Job drawing, mm, ordinate dimensions from the low corner. One solid piece. Coordinates: 2 decimals unless noted, no trailing zeros. Loops run counter-clockwise (first coordinate to the right, second up) from the corner with the lowest first, then second, coordinate; pieces in that order, holes last. Notation, with made-up numbers: (17.25, 45.5) - (73.25, 45.5) arc R27 ccw to (73.25, 82.5) - close; hole circle Ø1 at (58.5, -7). An arc over 180 degrees is marked (long way). Use a Markdown table: item, result. Add a question column.
1. Band-saw the part on A-A, the plane y = 25.4. Give the cut face in (x, z), plus the area to 3 significant figures.
2. Band-saw the part on B-B, the plane z = 12.7. Give the cut face in (x, y), plus the area to 3 significant figures.
3. Wall check: probe 1 along Y at (x, z) = (2.75, 12.7); probe 2 along Y at (x, z) = (2, 38.1); probe 3 along Z at (x, y) = (2, 25). Give the ranges that are in metal, low to high. Write a range as [from, to].
4. Pull direction Z, two halves, no side cores. Call the marked faces 1, 2 and 3: pulls with the +Z half, pulls with the -Z half, needs draft (parallel to the pull), parting line crosses it, or undercut.
5. Band-saw the part on C-C, the plane z = 32. Give the cut face in (x, y), plus the area to 3 significant figures.
6. Band-saw the part on D-D, the plane z = 57.5. Give the cut face in (x, y).
7. Drop flat-ended pins along their axis: pin 1 (2 mm diameter, centred on x = 3.5, y = 10, fed in from -Z); pin 2 (4 mm diameter, centred on y = 9.525, z = 12.7, fed in from +X). Give the stop position or say it passes through.
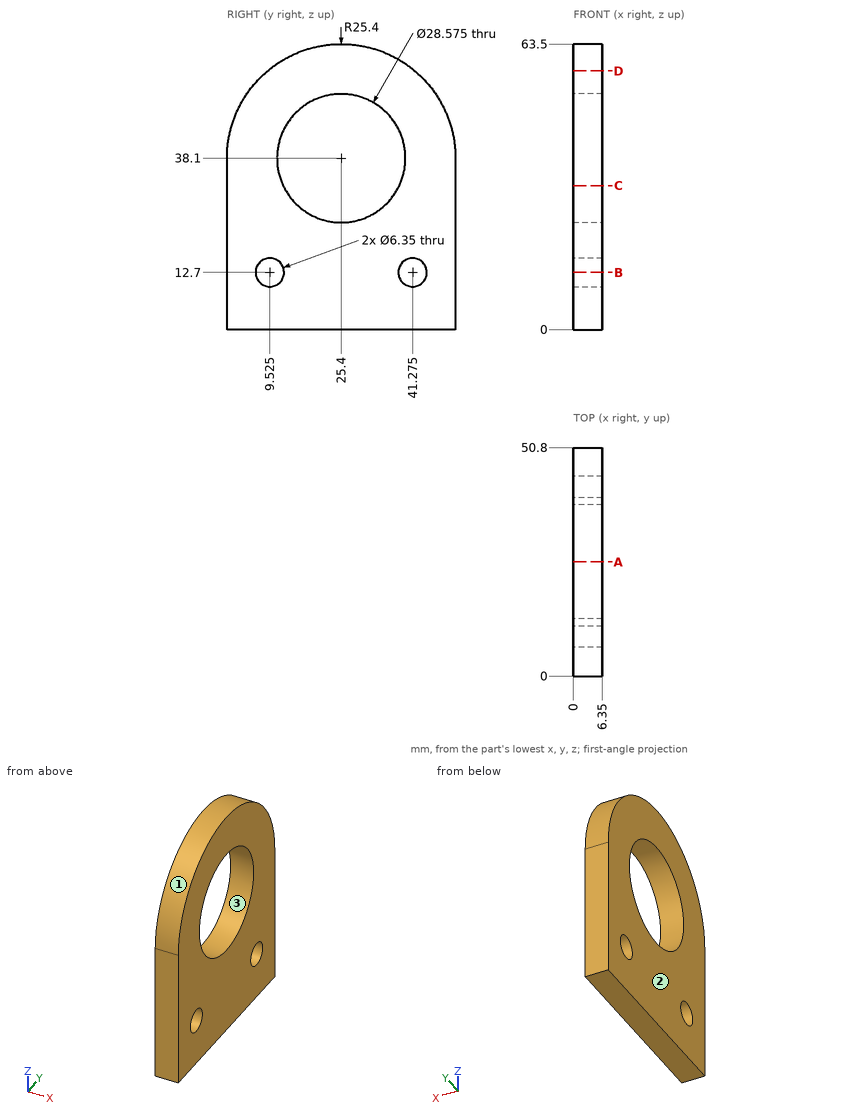
Geometry check:
| question | item | result |
|---|---|---|
| 1 | outline | (0, 0) - (6.35, 0) - (6.35, 23.81) - (0, 23.81) - close; (0, 52.39) - (6.35, 52.39) - (6.35, 63.5) - (0, 63.5) - close |
| 1 | area | 222 mm^2 |
| 2 | outline | (0, 0) - (6.35, 0) - (6.35, 6.35) - (0, 6.35) - close; (0, 12.7) - (6.35, 12.7) - (6.35, 38.1) - (0, 38.1) - close; (0, 44.45) - (6.35, 44.45) - (6.35, 50.8) - (0, 50.8) - close |
| 2 | area | 242 mm^2 |
| 3 | probe 1 | y = [0, 6.35], [12.7, 38.1], [44.45, 50.8] |
| 3 | probe 2 | y = [0, 11.11], [39.69, 50.8] |
| 3 | probe 3 | z = [0, 23.82], [52.38, 63.5] |
| 4 | face 1 | pulls with the +Z half |
| 4 | face 2 | needs draft |
| 4 | face 3 | undercut |
| 5 | outline | (0, 0) - (6.35, 0) - (6.35, 12.48) - (0, 12.48) - close; (0, 38.32) - (6.35, 38.32) - (6.35, 50.8) - (0, 50.8) - close |
| 5 | area | 158 mm^2 |
| 6 | outline | (0, 9) - (6.35, 9) - (6.35, 41.8) - (0, 41.8) - close |
| 7 | pin 1 | stops at z = 0 |
| 7 | pin 2 | passes through |
